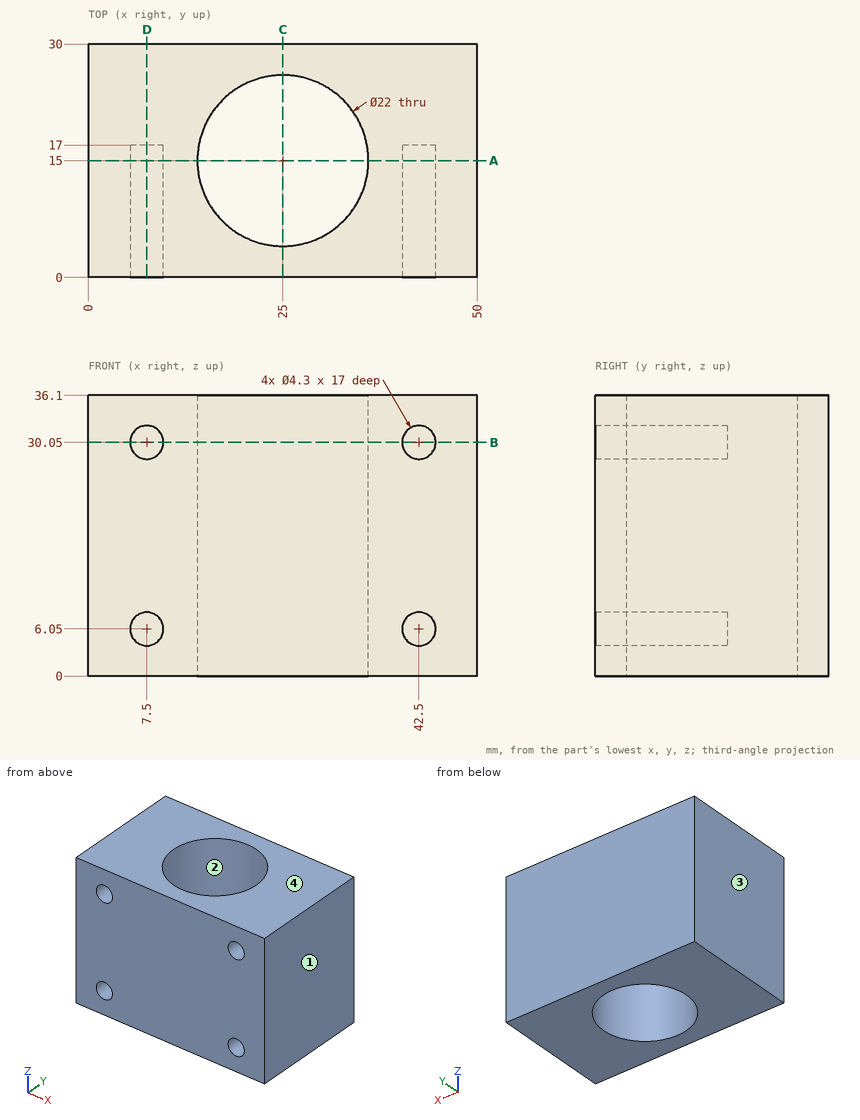
Verification items for this drawing (mm, ordinates from the low corner). Coordinates: 2 decimals unless noted, no trailing zeros. Write each loop counter-clockwise with the first axis right and the second up, starting at its lowest first coordinate (ties: lowest second). Pieces come first, ordered by that corner, then holes. Notation, with made-up numbers: M 4.5,-29.5 L 17.5,-29.5 A35 ccw 17.5,2.5 Z; hole C -14,39.5 d5. An arc over 180 degrees is marked long. Answer as a JSON object with one key per item and string values.
1. Section check C-C, the plane x = 25. Enter the section's corners in (y, z), plus the area to 3 significant figures.
Answers below:
{"outline": "M 0,0 L 4,0 L 4,36.1 L 0,36.1 Z; M 26,0 L 30,0 L 30,36.1 L 26,36.1 Z", "area": "289 mm²"}
2. Scan lines: L1, parallel to Z at x = 42.5, y = 5.75; L2, parallel to Y at x = 25.5, z = 19; L3, parallel to Y at x = 17, z = 3. Record each from-to range of solid material in increasing order.
Answers below:
{"L1": "z = 0 to 3.9, 8.2 to 27.9, 32.2 to 36.1", "L2": "y = 0 to 4.01, 25.99 to 30", "L3": "y = 0 to 7.45, 22.55 to 30"}
3. Section check D-D, the plane x = 7.5. Enter the section's corners in (y, z), plus the area to 3 significant figures.
Answers below:
{"outline": "M 0,0 L 30,0 L 30,36.1 L 0,36.1 L 0,32.2 L 17,32.2 L 17,27.9 L 0,27.9 L 0,8.2 L 17,8.2 L 17,3.9 L 0,3.9 Z", "area": "937 mm²"}
4. Go/stop test with flat-tipped pins: pin 1 Ø6 at (x, y) = (24.5, 20.5) entering from +Z; pin 2 Ø8 at (x, y) = (11.5, 10) entering from -Z; pin 3 Ø2 at (x, z) = (7.5, 5.5) entering from -Y. Record where each tip stops, or that it passes through.
Answers below:
{"pin 1": "passes through", "pin 2": "stops at z = 0", "pin 3": "stops at y = 17"}
5. Section check B-B, the plane z = 30.05. Enter the section's corners in (x, y), plus the area to 3 significant figures.
Answers below:
{"outline": "M 0,0 L 5.35,0 L 5.35,17 L 9.65,17 L 9.65,0 L 40.35,0 L 40.35,17 L 44.65,17 L 44.65,0 L 50,0 L 50,30 L 0,30 Z; hole C 25,15 d22", "area": "974 mm²"}
6. Section check A-A, the plane y = 15. Enter the section's corners in (x, z).
Answers below:
{"outline": "M 0,0 L 14,0 L 14,36.1 L 0,36.1 Z; M 36,0 L 50,0 L 50,36.1 L 36,36.1 Z; hole C 7.5,6.05 d4.3; hole C 7.5,30.05 d4.3; hole C 42.5,6.05 d4.3; hole C 42.5,30.05 d4.3"}
7. Draft check along X on the marked faces 1, 2, 3 and 4. Enter one of: released by +X, released by -X, zero draft, split by the parting line, or undercut.
Answers below:
{"face 1": "released by +X", "face 2": "undercut", "face 3": "released by -X", "face 4": "zero draft"}
